The listing builds one solid part. Answer for the finished solid, in the listing's coordinates (mm). A direction names the side the tool comes from. Give positions to 0.01 mm unless a question says otherwise; leave off trailing zeros. Order: outer loops, then holes, each group sorted by start corner. A loop starts at its lowest first (then second) coordinate and runs counter-clockwise, first axis right, second up. Notation, with made-up numbers: (37.25, 1.5) - (95.25, 1.5) arc R21 cw to (95.25, 26.5) - close; hole circle Ø9 at (69.25, 24.5). An arc over 180 degrees is marked (long way). Answer in a Markdown table with one row per item.
from build123d import *

# Parameters (mm, degrees)
ESQUISSE2_W             = 30.5
ESQUISSE2_H             = 18
BOSS_EXTRU_1_DEPTH      = 10
ESQUISSE3_W             = 8.5
ESQUISSE3_H             = 7
ENL_V_MAT_EXTRU_1_DEPTH = 3.4
ENL_V_MAT_EXTRU_2_DEPTH = 19.897685043
ESQUISSE7_W             = 8.5
ESQUISSE7_H             = 4
ENL_V_MAT_EXTRU_4_DEPTH = 1.9
CONG_1_R                = 3
ESQUISSE5_R             = 6
ESQUISSE5_R_2           = 3
ESQUISSE5_R_3           = 1.5
ENL_V_MAT_EXTRU_3_DEPTH = 0.1
ESQUISSE6_R             = 2
BOSS_EXTRU_2_DEPTH      = 20


with BuildPart() as part:
    # Esquisse2 → Boss.-Extru.1 (new body)
    with BuildSketch(Plane(origin=(0, 0, 0), x_dir=(1, 0, 0), z_dir=(0, 1, 0))):
        Rectangle(ESQUISSE2_W, ESQUISSE2_H)
    extrude(amount=BOSS_EXTRU_1_DEPTH)

    # Esquisse3 → Enlèv. mat.-Extru.1 (cut)
    with BuildSketch(Plane(origin=(0, 10, 0), x_dir=(1, 0, 0), z_dir=(0, 1, 0))):
        with Locations((11, -5.5)):
            Rectangle(ESQUISSE3_W, ESQUISSE3_H)
        with Locations((11, 5.5)):
            Rectangle(ESQUISSE3_W, ESQUISSE3_H)
    extrude(amount=-ENL_V_MAT_EXTRU_1_DEPTH, mode=Mode.SUBTRACT)

    # Esquisse4 → Enlèv. mat.-Extru.2 (cut, through all)
    with BuildSketch(Plane(origin=(0, 6.6, 0), x_dir=(1, 0, 0), z_dir=(0, 1, 0))):
        with BuildLine():
            Line((10, 7.75), (11.5, 7.75))
            ThreePointArc((11.5, 7.75), (13.25, 6), (11.5, 4.25))
            Line((11.5, 4.25), (10, 4.25))
            ThreePointArc((10, 4.25), (8.25, 6), (10, 7.75))
        make_face()
        with BuildLine():
            Line((10, -7.75), (11.5, -7.75))
            ThreePointArc((11.5, -7.75), (13.25, -6), (11.5, -4.25))
            Line((11.5, -4.25), (10, -4.25))
            ThreePointArc((10, -4.25), (8.25, -6), (10, -7.75))
        make_face()
    extrude(amount=-ENL_V_MAT_EXTRU_2_DEPTH, mode=Mode.SUBTRACT)

    # Esquisse7 → Enlèv. mat.-Extru.4 (cut)
    with BuildSketch(Plane(origin=(0, 10, 0), x_dir=(1, 0, 0), z_dir=(0, 1, 0))):
        with Locations((11, 0)):
            Rectangle(ESQUISSE7_W, ESQUISSE7_H)
    extrude(amount=-ENL_V_MAT_EXTRU_4_DEPTH, mode=Mode.SUBTRACT)

    # Congé1
    cong_1_edges = [part.edges().sort_by_distance(p)[0] for p in [
        (6.75, 7.35, 2),
        (6.75, 7.35, -2),
    ]]
    fillet(cong_1_edges, radius=CONG_1_R)

    # Esquisse5 → Enlèv. mat.-Extru.3 (cut)
    # profile 1 of 2: a face of its own
    with BuildSketch(Plane(origin=(0, 10, 0), x_dir=(1, 0, 0), z_dir=(0, 1, 0))):
        with Locations(Location((-7.25, 0, 0), (0, 0, 270))):
            Circle(ESQUISSE5_R)
        with Locations(Location((-7.25, 0, 0), (0, 0, 270))):
            Circle(ESQUISSE5_R_2, mode=Mode.SUBTRACT)
    # profile 2 of 2: a face of its own
    with BuildSketch(Plane(origin=(0, 10, 0), x_dir=(1, 0, 0), z_dir=(0, 1, 0))):
        with Locations(Location((2.75, -5, 0), (0, 0, 270))):
            Circle(ESQUISSE5_R_3)
    extrude(amount=-ENL_V_MAT_EXTRU_3_DEPTH, mode=Mode.SUBTRACT)

    # Esquisse6 → Boss.-Extru.2 (add)
    with BuildSketch(Plane(origin=(15.25, 0, 0), x_dir=(0, 0, -1), z_dir=(1, 0, 0))):
        with Locations(Location((0, 3.5, 0), (0, 0, 180))):
            Circle(ESQUISSE6_R)
    extrude(amount=BOSS_EXTRU_2_DEPTH)


solid = part.part
Item 1: Which of the six approach directions +Z, -Z, +X, -X, +Y, -Y give full straight-line access (tool end or side, diameter ignored) to faces 4 (the face through (11, 3, 7.75)), 5 (the face through (10, 8.1, 0)), 6 (the face through (25.11, 5.452, -0.434))?
Answer block:
| item | result |
|---|---|
| face 4 | +Y, -Y |
| face 5 | +Z, -Z, +X, +Y |
| face 6 | +X |
Item 2: Find section A-A on x = 10.5. Write down the section's boundary in (y, z), then the cut area to 3 significant figures.
Answer block:
| item | result |
|---|---|
| outline | (0, -9) - (6.6, -9) - (6.6, -7.75) - (0, -7.75) - close; (0, -4.25) - (6.6, -4.25) - (6.6, -2) - (8.1, -2) - (8.1, 2) - (6.6, 2) - (6.6, 4.25) - (0, 4.25) - close; (0, 7.75) - (6.6, 7.75) - (6.6, 9) - (0, 9) - close |
| area | 78.6 mm² |
Item 3: Find section B-B on y = 3.5. Write down the section's boundary in (x, z), then the cut area to 3 significant figures.
Answer block:
| item | result |
|---|---|
| outline | (-15.25, -9) - (15.25, -9) - (15.25, -2) - (35.25, -2) - (35.25, 2) - (15.25, 2) - (15.25, 9) - (-15.25, 9) - close; hole (10, -7.75) - (11.5, -7.75) arc R1.75 ccw to (11.5, -4.25) - (10, -4.25) arc R1.75 ccw to start; hole (10, 4.25) - (11.5, 4.25) arc R1.75 ccw to (11.5, 7.75) - (10, 7.75) arc R1.75 ccw to start |
| area | 599 mm² |
Item 4: Consider line 1 (X direction, y = 9.95, z = 0); line 2 (X direction, y = 6, z = 6); line 3 (X direction, y = 7.5, z = 1.5). Determine where each line is inside the solid, lowest interval first.
Answer block:
| item | result |
|---|---|
| line 1 | -15.25 to -13.25, -10.25 to -4.25, -1.25 to 6.75 |
| line 2 | -15.25 to 8.25, 13.25 to 15.25 |
| line 3 | -15.25 to 15.25 |
Item 5: Determine the mould class of faces 1 (the face through (3, 9.9, 5)), 2 (the face through (12, 7, 2)), 3 (the face through (-7, 10, 0)) for opening direction Z: pulls with the +Z half, pulls with the -Z half, needs draft (parallel to the pull), parting line crosses it, or undercut.
Answer block:
| item | result |
|---|---|
| face 1 | undercut |
| face 2 | pulls with the +Z half |
| face 3 | needs draft |
Item 6: Each of these flat-tipped pins is pushed along its axis until it touches: P1, Ø2, axis at x = 11, z = -5, coming from the +Y side; P2, Ø2, axis at x = 11.5, z = 6, coming from the +Y side; P3, Ø0.8, axis at x = 11.5, y = 7.5, coming from the +Z side; P4, Ø0.8, axis at x = 11, y = 7.5, coming from the -Z side. Where does it stop, or does it pass through?
Answer block:
| item | result |
|---|---|
| P1 | y = 6.6 |
| P2 | through |
| P3 | z = 2 |
| P4 | z = -2 |
Item 7: Find section C-C on y = 9. Write down the section's boundary in (x, z).
Answer block:
| item | result |
|---|---|
| outline | (-15.25, -9) - (6.75, -9) - (6.75, 9) - (-15.25, 9) - close |
